Could you check a few things on this model? Use its own coordinates, in mm. Face numbers are marked on the shaded views. A direction names the side the tool comes from. Coordinates: 2 decimals unless noted, no trailing zeros. Write each loop counter-clockwise with the first axis right and the second up, starting at its lowest first coordinate (ties: lowest second). Pieces come first, ordered by that corner, then holes. Notation, with made-up numbers: (3, 7.5) - (42, 7.5) arc R21 ccw to (42, 38.5) - close; hole circle Ø3 at (19, 36). An arc over 180 degrees is marked (long way). Answer as a JSON object with one key per item and string values. Group by question number.
1) Will these pins go through, and if not, where does the flat tip stop? pin 1 Ø1.5 at (x, y) = (3.5, -2) entering from -Z; pin 2 Ø1.6 at (y, z) = (-1.5, 8) entering from -X; pin 3 Ø2 at (x, y) = (9.5, -1.5) entering from +Z.
2) On a 3-axis mill with a long thin cutter (end or side, diameter ignored), from which of +Z, -Z, +X, -X, +Y, -Y can I reach the whole of each face in a straight line? I mean the marked faces 1, 2, 3 and 4. Say none if no direction works.
3) Please list where these lines run through material, in increasing order: line 1 along X through (y, z) = (-1.15, 9); line 2 along X through (y, z) = (-0.65, 5.5); line 3 along Z through (x, y) = (7.75, -1.8).
4) We'd pull the mould along Z, two halves only. Please class the marked faces 5, 6 and 7: released by +Z, released by -Z, zero draft, split by the parting line, or undercut.
5) If we section it at D-D (y = 0.35): Write out the boundary of the cut face in (x, z).
6) If we section it at A-A (y = -1.35): Write out the boundary of the cut face in (x, z).
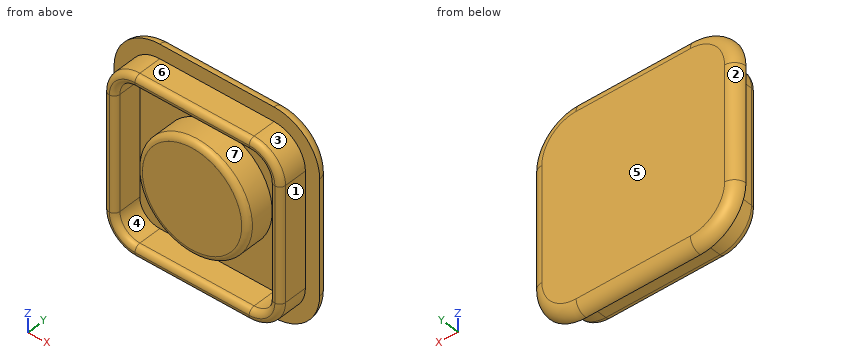
```python
from build123d import *

# Parameters (mm, degrees)
SKETCH1_W           = 18
SKETCH1_H           = 18
BOSS_EXTRUDE1_DEPTH = 1
FILLET1_R           = 4
SKETCH2_R           = 4.85
SKETCH2_R_2         = 3.85
BOSS_EXTRUDE2_DEPTH = 2.5
FILLET2_R           = 1
FILLET3_R           = 0.5


with BuildPart() as part:
    # Sketch1 → Boss-Extrude1 (new body)
    with BuildSketch(Plane(origin=(0, 0, 0), x_dir=(1, 0, 0), z_dir=(0, 1, 0))):
        with Locations((9, -9)):
            Rectangle(SKETCH1_W, SKETCH1_H)
    extrude(amount=BOSS_EXTRUDE1_DEPTH)

    # Fillet1
    fillet1_edges = [part.edges().sort_by_distance(p)[0] for p in [
        (0, 0.5, 0),
        (18, 0.5, 0),
        (18, 0.5, 18),
        (0, 0.5, 18),
    ]]
    fillet(fillet1_edges, radius=FILLET1_R)

    # Sketch2 → Boss-Extrude2 (add)
    # profile 1 of 2: a face of its own
    with BuildSketch(Plane.XZ):
        with BuildLine():
            Line((1.25, 14), (1.25, 4))
            ThreePointArc((1.25, 4), (2.055456352, 2.055456352), (4, 1.25))
            Line((4, 1.25), (14, 1.25))
            ThreePointArc((14, 1.25), (15.944543648, 2.055456352), (16.75, 4))
            Line((16.75, 4), (16.75, 14))
            ThreePointArc((16.75, 14), (15.944543648, 15.944543648), (14, 16.75))
            Line((14, 16.75), (4, 16.75))
            ThreePointArc((4, 16.75), (2.055456352, 15.944543648), (1.25, 14))
        make_face()
        with BuildLine():
            Line((2.25, 14), (2.25, 4))
            ThreePointArc((2.25, 4), (2.762563133, 2.762563133), (4, 2.25))
            Line((4, 2.25), (14, 2.25))
            ThreePointArc((14, 2.25), (15.237436867, 2.762563133), (15.75, 4))
            Line((15.75, 4), (15.75, 14))
            ThreePointArc((15.75, 14), (15.237436867, 15.237436867), (14, 15.75))
            Line((14, 15.75), (4, 15.75))
            ThreePointArc((4, 15.75), (2.762563133, 15.237436867), (2.25, 14))
        make_face(mode=Mode.SUBTRACT)
    # profile 2 of 2: a face of its own
    with BuildSketch(Plane.XZ):
        with Locations(Location((9, 9, 0), (0, 0, 90))):
            Circle(SKETCH2_R)
        with Locations(Location((9, 9, 0), (0, 0, 270))):
            Circle(SKETCH2_R_2, mode=Mode.SUBTRACT)
    extrude(amount=BOSS_EXTRUDE2_DEPTH)

    # Fillet2
    fillet2_edges = [part.edges().sort_by_distance(p)[0] for p in [
        (16.828427125, 1, 1.171572875),
        (18, 1, 9),
        (16.828427125, 1, 16.828427125),
        (9, 1, 18),
        (1.171572875, 1, 16.828427125),
        (0, 1, 9),
        (1.171572875, 1, 1.171572875),
        (9, 1, 0),
    ]]
    fillet(fillet2_edges, radius=FILLET2_R - 0.0001)  # a hair under: the kernel refuses the full size

    # Fillet3
    fillet3_edges = [part.edges().sort_by_distance(p)[0] for p in [
        (2.762563133, -2.5, 15.237436867),
        (9, -2.5, 15.75),
        (15.237436867, -2.5, 15.237436867),
        (15.75, -2.5, 9),
        (15.237436867, -2.5, 2.762563133),
        (9, -2.5, 2.25),
        (2.762563133, -2.5, 2.762563133),
        (2.25, -2.5, 9),
        (9, -2.5, 16.75),
        (2.055456352, -2.5, 15.944543648),
        (1.25, -2.5, 9),
        (2.055456352, -2.5, 2.055456352),
        (9, -2.5, 1.25),
        (15.944543648, -2.5, 2.055456352),
        (16.75, -2.5, 9),
        (15.944543648, -2.5, 15.944543648),
        (9, -2.5, 12.85),
        (9, -2.5, 4.15),
    ]]
    fillet(fillet3_edges, radius=FILLET3_R - 0.0001)  # a hair under: the kernel refuses the full size


solid = part.part
```
Here are the results:
{
 "1": {"pin 1": "stops at z = 1.25", "pin 2": "stops at x = 1.25", "pin 3": "stops at z = 16.75"},
 "2": {"face 1": "+Z, -Z, +X, -Y", "face 2": "+Z, -Z, -X, +Y", "face 3": "+Z, +X, -Y", "face 4": "-Y"},
 "3": {"line 1": "x = 1.25 to 2.25, 4.15 to 5.15, 12.85 to 13.85, 15.75 to 16.75", "line 2": "x = 1.25 to 2.25, 5.64 to 7.4, 10.6 to 12.36, 15.75 to 16.75", "line 3": "z = 1.25 to 2.25, 4.31 to 5.36, 12.64 to 13.69, 15.75 to 16.75"},
 "4": {"face 5": "zero draft", "face 6": "released by +Z", "face 7": "undercut"},
 "5": {"outline": "(0.06, 4) arc R3.94 ccw to (4, 0.06) - (14, 0.06) arc R3.94 ccw to (17.94, 4) - (17.94, 14) arc R3.94 ccw to (14, 17.94) - (4, 17.94) arc R3.94 ccw to (0.06, 14) - close"},
 "6": {"outline": "(1.25, 4) arc R2.75 ccw to (4, 1.25) - (14, 1.25) arc R2.75 ccw to (16.75, 4) - (16.75, 14) arc R2.75 ccw to (14, 16.75) - (4, 16.75) arc R2.75 ccw to (1.25, 14) - close; circle Ø9.7 at (9, 9); hole (2.25, 4) arc R1.75 ccw to (4, 2.25) - (14, 2.25) arc R1.75 ccw to (15.75, 4) - (15.75, 14) arc R1.75 ccw to (14, 15.75) - (4, 15.75) arc R1.75 ccw to (2.25, 14) - close; hole circle Ø7.7 at (9, 9)"}
}
